Here's how the part is built. I have some questions about the finished solid (model axes, mm). A direction names the side the tool comes from. Give positions to 0.01 mm unless a question says otherwise; leave off trailing zeros. Loops run counter-clockwise (first coordinate to the right, second up) from the corner with the lowest first, then second, coordinate; pieces in that order, holes last. Notation, with made-up numbers: (-2, 46) - (38, 46) arc R20 cw to (38, 60) - close; hole circle Ø10 at (71.5, 24.25). An arc over 180 degrees is marked (long way). Use a Markdown table: item, result.
from build123d import *

# Parameters (mm, degrees)
SKETCH1_R           = 10
BOSS_EXTRUDE1_DEPTH = 25.4
CUT_EXTRUDE1_REACH  = 101.47
SKETCH2_R           = 2.7432
SKETCH2_R_2         = 2.54
CUT_EXTRUDE2_DEPTH  = 12.7
FILLET1_R           = 1.016


with BuildPart() as part:
    # Sketch1 → Boss-Extrude1 (new body)
    with BuildSketch(Plane.XY):
        Polygon((-58.674, 12.7), (-33.274, 12.7), (-33.274, -50.8), (-20.574, -50.8), (-20.574, -25.4), (19.05, -25.4), (19.05, 25.4), (-58.674, 25.4), align=None)
        Circle(SKETCH1_R, mode=Mode.SUBTRACT)
    extrude(amount=BOSS_EXTRUDE1_DEPTH)

    # Sketch2 → Cut-Extrude1 (cut, up to next)
    with BuildSketch(Plane(origin=(0, 25.4, 0), x_dir=(1, 0, 0), z_dir=(0, 1, 0)), mode=Mode.PRIVATE) as cut_extrude1_sk1:
        with Locations(Location((-45.974, -12.7, 0), (0, 0, 180))):
            Circle(SKETCH2_R)
    cut_extrude1_tool1 = extrude(cut_extrude1_sk1.sketch, amount=-CUT_EXTRUDE1_REACH, mode=Mode.PRIVATE) & part.part
    # Sketch2 → Cut-Extrude1 (cut, up to next)
    with BuildSketch(Plane(origin=(0, 25.4, 0), x_dir=(1, 0, 0), z_dir=(0, 1, 0)), mode=Mode.PRIVATE) as cut_extrude1_sk2:
        with Locations(Location((0, -12.7, 0), (0, 0, 180))):
            Circle(SKETCH2_R_2)
    cut_extrude1_tool2 = extrude(cut_extrude1_sk2.sketch, amount=-CUT_EXTRUDE1_REACH, mode=Mode.PRIVATE) & part.part
    add(cut_extrude1_tool1.solids().sort_by_distance((-45.974, 25.4, 12.7))[0], mode=Mode.SUBTRACT)
    add(cut_extrude1_tool2.solids().sort_by_distance((0, 25.4, 12.7))[0], mode=Mode.SUBTRACT)

    # Sketch3 → Cut-Extrude2 (cut)
    with BuildSketch(Plane(origin=(-20.574, 0, 0), x_dir=(0, 0, -1), z_dir=(1, 0, 0))):
        with BuildLine():
            Line((-9.9568, -34.925), (-9.9568, -41.275))
            ThreePointArc((-9.9568, -41.275), (-12.7, -44.0182), (-15.4432, -41.275))
            Line((-15.4432, -41.275), (-15.4432, -34.925))
            ThreePointArc((-15.4432, -34.925), (-12.7, -32.1818), (-9.9568, -34.925))
        make_face()
    extrude(amount=-CUT_EXTRUDE2_DEPTH, mode=Mode.SUBTRACT)

    # Fillet1
    fillet1_edges = [part.edges().sort_by_distance(p)[0] for p in [
        (-20.574, -25.4, 12.7),
        (-33.274, 12.7, 12.7),
    ]]
    fillet(fillet1_edges, radius=FILLET1_R)


solid = part.part
(1) Suppose I cut it at B-B on z = 20.75. Write out the boundary of the cut face in (x, y), plus the area to 3 significant figures.
A:
| item | result |
|---|---|
| outline | (-58.67, 12.7) - (-34.29, 12.7) arc R1.02 cw to (-33.27, 11.68) - (-33.27, -50.8) - (-20.57, -50.8) - (-20.57, -26.42) arc R1.02 cw to (-19.56, -25.4) - (19.05, -25.4) - (19.05, 25.4) - (-58.67, 25.4) - close; hole circle Ø20 at (0, 0) |
| area | 2,990 mm2 |
(2) Suppose I cut it at D-D on z = 12.7. Write out the boundary of the cut face in (x, y).
A:
| item | result |
|---|---|
| outline | (-58.67, 12.7) - (-48.72, 12.7) - (-48.72, 25.4) - (-58.67, 25.4) - close; (-43.23, 12.7) - (-34.29, 12.7) arc R1.02 cw to (-33.27, 11.68) - (-33.27, -32.18) - (-20.57, -32.18) - (-20.57, -26.42) arc R1.02 cw to (-19.56, -25.4) - (19.05, -25.4) - (19.05, 25.4) - (2.54, 25.4) - (2.54, 9.67) arc R10 cw (long way) to (-2.54, 9.67) - (-2.54, 25.4) - (-43.23, 25.4) - close; (-33.27, -50.8) - (-20.57, -50.8) - (-20.57, -44.02) - (-33.27, -44.02) - close |
(3) Will these pins go through, and if not, where does the flat tip stop? pin 1 (12 mm diameter, centred on x = -52.5, z = 16, fed in from -Y); pin 2 (12.5 mm diameter, centred on y = -34.5, z = 10, fed in from -X); pin 3 (8 mm diameter, centred on x = 0, z = 12.7, fed in from -Y).
A:
| item | result |
|---|---|
| pin 1 | y = 12.7 |
| pin 2 | x = -33.27 |
| pin 3 | y = -25.4 |
(4) If I drill on line 1 (X direction, y = 0.5, z = 19.25); line 2 (Z direction, x = 0, y = 15.5); line 3 (Y direction, x = -35.5, z = 8.25), over which ranges is the centre line in solid material (lowest first)?
A:
| item | result |
|---|---|
| line 1 | -33.27 to -9.99, 9.99 to 19.05 |
| line 2 | 0 to 10.16, 15.24 to 25.4 |
| line 3 | 12.7 to 25.4 |
(5) Suppose I cut it at C-C on y = 0. Write out the boundary of the cut face in (x, z).
A:
| item | result |
|---|---|
| outline | (-33.27, 0) - (-10, 0) - (-10, 25.4) - (-33.27, 25.4) - close; (10, 0) - (19.05, 0) - (19.05, 25.4) - (10, 25.4) - close |
(6) We'd pull the mould along X, two halves only. Please class faces 5 (the face through (-43.233, 19.139, 12.821)), 6 (the face through (-20.574, -38.8, 9.7)), 7 (the face through (-12, -4, 25.4)): pulls with the +X half, pulls with the -X half, needs draft (parallel to the pull), parting line crosses it, or undercut.
A:
| item | result |
|---|---|
| face 5 | undercut |
| face 6 | pulls with the +X half |
| face 7 | needs draft |
(7) Suppose I cut it at A-A on x = 0. Write out the boundary of the cut face in (y, z), plus the area to 3 significant figures.
A:
| item | result |
|---|---|
| outline | (-25.4, 0) - (-10, 0) - (-10, 25.4) - (-25.4, 25.4) - close; (10, 0) - (25.4, 0) - (25.4, 10.16) - (10, 10.16) - close; (10, 15.24) - (25.4, 15.24) - (25.4, 25.4) - (10, 25.4) - close |
| area | 704 mm2 |
(8) On a 3-axis mill with a long thin cutter (end or side, diameter ignored), from which of +Z, -Z, +X, -X, +Y, -Y can I reach the whole of each face in a straight line? I mean faces 1 (the face through (-1, -25.4, 13)), 2 (the face through (-33.274, -19, 13)), 3 (the face through (-27, -38, 9.957)), 4 (the face through (0.33, 17.64, 15.22)). Say none if no direction works.
A:
| item | result |
|---|---|
| face 1 | +Z, -Z, +X, -Y |
| face 2 | +Z, -Z, -X, -Y |
| face 3 | +X, -X |
| face 4 | +Y |
